Design review of the part shown in the three views and the two pictorial views. Dimensions are in mm from the part's minimum x, y and z. A direction names the side the tool comes from. Coordinates: 2 decimals unless noted, no trailing zeros. Loops run counter-clockwise (first coordinate to the right, second up) from the corner with the lowest first, then second, coordinate; pieces in that order, holes last. Notation, with made-up numbers: M 17.5,2.25 L 47.5,2.25 A13 cw 47.5,9.25 Z; hole C 76,37 d2. An arc over 180 degrees is marked long. Use one line per item in the form item = value.
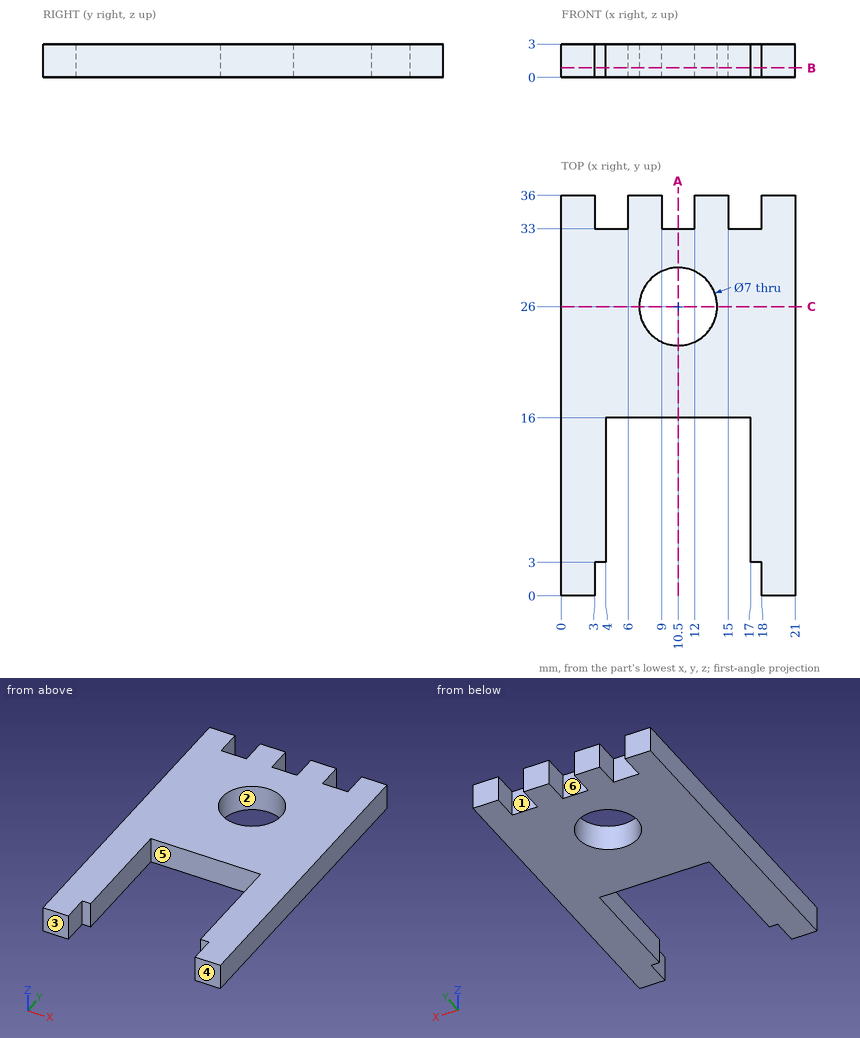
1. The part is to be moulded in two halves that separate along Y. For the marked faces 1, 2 and 3, say which applies: pulls with the +Y half, pulls with the -Y half, needs draft (parallel to the pull), parting line crosses it, or undercut.
Response values:
face_1 = pulls with the +Y half
face_2 = undercut
face_3 = pulls with the -Y half
2. Add section A-A (x = 10.5). State the section outline as (y, z) points, then the cut area to 3 significant figures.
Response values:
outline = M 16,0 L 22.5,0 L 22.5,3 L 16,3 Z; M 29.5,0 L 33,0 L 33,3 L 29.5,3 Z
area = 30.0 mm^2
3. Machinability: for the marked faces 4, 5 and 6, which of the approach directions +Z, -Z, +X, -X, +Y, -Y give a long, thin tool a straight path to every point of the face, cutting with its end or side? Answer none if there is none.
Response values:
face_4 = +Z, -Z, +X, -X, -Y
face_5 = +Z, -Z, -Y
face_6 = +Z, -Z, +Y
4. Wall thickness on line 1 along X through (y, z) = (6, 0.35); line 2 along Y through (x, z) = (10.5, 0.95); line 3 along Y through (x, z) = (8.25, 1.65): over which ranges is each line inside the solid? List them lowest first. Write a range as from..to.
Response values:
line_1 = 0..4, 17..21
line_2 = 16..22.5, 29.5..33
line_3 = 16..23.32, 28.68..36
5. Add section B-B (z = 0.85). State the section outline as (x, y) points, then the cut area to 3 significant figures.
Response values:
outline = M 0,0 L 3,0 L 3,3 L 4,3 L 4,16 L 17,16 L 17,3 L 18,3 L 18,0 L 21,0 L 21,36 L 18,36 L 18,33 L 15,33 L 15,36 L 12,36 L 12,33 L 9,33 L 9,36 L 6,36 L 6,33 L 3,33 L 3,36 L 0,36 Z; hole C 10.5,26 d7
area = 477 mm^2
6. Insertion check: P1, Ø0.8, axis at x = 17.5, z = 1, coming from the -Y side; P2, Ø1, axis at x = 6.5, z = 0.5, coming from the -Y side; P3, Ø5.5, axis at x = 10.5, y = 26, coming from the +Z side; P4, Ø0.9, axis at x = 4, z = 2, coming from the +Y side. Each pin has a flat end and moves straight along its axis. Give the tip position at first contact, or say it passes through.
Response values:
P1 = 3
P2 = 16
P3 = through
P4 = 33
7. Add section C-C (y = 26). State the section outline as (x, z) points, then the cut area to 3 significant figures.
Response values:
outline = M 0,0 L 7,0 L 7,3 L 0,3 Z; M 14,0 L 21,0 L 21,3 L 14,3 Z
area = 42.0 mm^2
